Read the model definition and answer for the solid it produces. Units are mm, in the model's axes. A direction names the side the tool comes from. Coordinates: 2 decimals unless noted, no trailing zeros. Order: outer loops, then holes, each group sorted by start corner. A loop starts at its lowest first (then second) coordinate and runs counter-clockwise, first axis right, second up. Notation, with made-up numbers: M -12.75,41.5 L 8.25,41.5 A15 ccw 8.25,54.5 Z; hole C 11,-19 d4. An arc over 180 degrees is marked long. Write each question's results on one line, items separated by ' | '.
```python
from build123d import *

# Parameters (mm, degrees)
PCB_DEPTH                       = 1.6
SKETCH2_W                       = 2
SKETCH2_H                       = 30
BODY00_DEPTH                    = 0.4
SKETCH3_W                       = 80.5
SKETCH3_H                       = 54.92
BODY01_DEPTH                    = 4.2
SKETCH4_W                       = 6
SKETCH4_H                       = 12
UNDER00_DEPTH                   = 5
SKETCH5_W                       = 15
SKETCH5_H                       = 11.5
UNDER01_DEPTH                   = 5.6
SKETCH6_W                       = 33.02
SKETCH6_H                       = 5.08
UNDER02_DEPTH                   = 8.5
SKETCH7_R                       = 2.5
SIDE0_AUDIO_JACK_NOSE_DEPTH     = 2.5
SKETCH8_R                       = 1.75
SIDEBORE0_AUDIO_JACK_NOSE_DEPTH = 2.5
SKETCH9_W                       = 14
SKETCH9_H                       = 4.5
CUT00_DEPTH                     = 11
SKETCH10_W                      = 1
SKETCH10_H                      = 1
CUT01_DEPTH                     = 8.5
SKETCH11_W                      = 73.44
SKETCH11_H                      = 48.96
CUT02_DEPTH                     = 0.2
SKETCH12_R                      = 1.375
HOLES_DEPTH                     = 1.6


with BuildPart() as part:
    # Sketch1 → PCB (new body)
    with BuildSketch(Plane.XY):
        with BuildLine():
            Line((1, 0), (84.42, 0))
            ThreePointArc((84.42, 0), (85.127106781, 0.292893219), (85.42, 1))
            Line((85.42, 1), (85.42, 54.92))
            ThreePointArc((85.42, 54.92), (85.127106781, 55.627106781), (84.42, 55.92))
            Line((84.42, 55.92), (1, 55.92))
            ThreePointArc((1, 55.92), (0.292893219, 55.627106781), (0, 54.92))
            Line((0, 54.92), (0, 1))
            ThreePointArc((0, 1), (0.292893219, 0.292893219), (1, 0))
        make_face()
    extrude(amount=PCB_DEPTH)

    # Sketch2 → Body00 (add)
    with BuildSketch(Plane.XY.offset(1.6)):
        with Locations((82.3, 35)):
            Rectangle(SKETCH2_W, SKETCH2_H)
    extrude(amount=BODY00_DEPTH)

    # Sketch3 → Body01 (add)
    with BuildSketch(Plane.XY.offset(1.6)):
        with Locations((40.75, 27.96)):
            Rectangle(SKETCH3_W, SKETCH3_H)
    extrude(amount=BODY01_DEPTH)

    # Sketch4 → Under00 (add)
    with BuildSketch(Plane.XY):
        with Locations((53.5, 6)):
            Rectangle(SKETCH4_W, SKETCH4_H)
    extrude(amount=-UNDER00_DEPTH)

    # Sketch5 → Under01 (add)
    with BuildSketch(Plane.XY):
        with Locations((32, 5.25)):
            Rectangle(SKETCH5_W, SKETCH5_H)
    extrude(amount=-UNDER01_DEPTH)

    # Sketch6 → Under02 (add)
    with BuildSketch(Plane.XY):
        with Locations((23.61, 52.5)):
            Rectangle(SKETCH6_W, SKETCH6_H)
    extrude(amount=-UNDER02_DEPTH)

    # Sketch7 → Side0_Audio_jack_nose (add)
    with BuildSketch(Plane(origin=(0, 0, 0), x_dir=(1, 0, 0), z_dir=(0, 1, 0))):
        with Locations(Location((53.5, 2.5, 0), (0, 0, 270))):
            Circle(SKETCH7_R)
    extrude(amount=-SIDE0_AUDIO_JACK_NOSE_DEPTH)

    # Sketch8 → SideBore0_Audio_jack_nose (cut)
    with BuildSketch(Plane(origin=(0, 0, 0), x_dir=(1, 0, 0), z_dir=(0, 1, 0))):
        with Locations(Location((53.5, 2.5, 0), (0, 0, 270))):
            Circle(SKETCH8_R)
    extrude(amount=-SIDEBORE0_AUDIO_JACK_NOSE_DEPTH, mode=Mode.SUBTRACT)

    # Sketch9 → Cut00 (cut)
    with BuildSketch(Plane(origin=(0, 10.5, 0), x_dir=(1, 0, 0), z_dir=(0, 1, 0))):
        with Locations((32, 2.8)):
            Rectangle(SKETCH9_W, SKETCH9_H)
    extrude(amount=-CUT00_DEPTH, mode=Mode.SUBTRACT)

    # Sketch10 → Cut01 (cut)
    with BuildSketch(Plane.XY):
        with Locations((8.37, 51.23)):
            Rectangle(SKETCH10_W, SKETCH10_H)
        with Locations((8.37, 53.77)):
            Rectangle(SKETCH10_W, SKETCH10_H)
        with Locations((10.91, 51.23)):
            Rectangle(SKETCH10_W, SKETCH10_H)
        with Locations((10.91, 53.77)):
            Rectangle(SKETCH10_W, SKETCH10_H)
        with Locations((13.45, 51.23)):
            Rectangle(SKETCH10_W, SKETCH10_H)
        with Locations((13.45, 53.77)):
            Rectangle(SKETCH10_W, SKETCH10_H)
        with Locations((15.99, 51.23)):
            Rectangle(SKETCH10_W, SKETCH10_H)
        with Locations((15.99, 53.77)):
            Rectangle(SKETCH10_W, SKETCH10_H)
        with Locations((18.53, 51.23)):
            Rectangle(SKETCH10_W, SKETCH10_H)
        with Locations((18.53, 53.77)):
            Rectangle(SKETCH10_W, SKETCH10_H)
        with Locations((21.07, 51.23)):
            Rectangle(SKETCH10_W, SKETCH10_H)
        with Locations((21.07, 53.77)):
            Rectangle(SKETCH10_W, SKETCH10_H)
        with Locations((23.61, 51.23)):
            Rectangle(SKETCH10_W, SKETCH10_H)
        with Locations((23.61, 53.77)):
            Rectangle(SKETCH10_W, SKETCH10_H)
        with Locations((26.15, 51.23)):
            Rectangle(SKETCH10_W, SKETCH10_H)
        with Locations((26.15, 53.77)):
            Rectangle(SKETCH10_W, SKETCH10_H)
        with Locations((28.69, 51.23)):
            Rectangle(SKETCH10_W, SKETCH10_H)
        with Locations((28.69, 53.77)):
            Rectangle(SKETCH10_W, SKETCH10_H)
        with Locations((31.23, 51.23)):
            Rectangle(SKETCH10_W, SKETCH10_H)
        with Locations((31.23, 53.77)):
            Rectangle(SKETCH10_W, SKETCH10_H)
        with Locations((33.77, 51.23)):
            Rectangle(SKETCH10_W, SKETCH10_H)
        with Locations((33.77, 53.77)):
            Rectangle(SKETCH10_W, SKETCH10_H)
        with Locations((36.31, 51.23)):
            Rectangle(SKETCH10_W, SKETCH10_H)
        with Locations((36.31, 53.77)):
            Rectangle(SKETCH10_W, SKETCH10_H)
        with Locations((38.85, 51.23)):
            Rectangle(SKETCH10_W, SKETCH10_H)
        with Locations((38.85, 53.77)):
            Rectangle(SKETCH10_W, SKETCH10_H)
    extrude(amount=-CUT01_DEPTH, mode=Mode.SUBTRACT)

    # Sketch11 → Cut02 (cut)
    with BuildSketch(Plane.XY.offset(5.8)):
        with Locations((40, 27.96)):
            Rectangle(SKETCH11_W, SKETCH11_H)
    extrude(amount=-CUT02_DEPTH, mode=Mode.SUBTRACT)

    # Sketch12 → Holes (cut)
    with BuildSketch(Plane.XY.offset(1.6)):
        with Locations((3.5, 3.5)):
            Circle(SKETCH12_R)
        with Locations((3.5, 52.5)):
            Circle(SKETCH12_R)
        with Locations((61.5, 3.5)):
            Circle(SKETCH12_R)
        with Locations((61.5, 52.5)):
            Circle(SKETCH12_R)
    extrude(amount=-HOLES_DEPTH, mode=Mode.SUBTRACT)


solid = part.part
```
(1) The mould has two halves that part along Y. Classify faces 6 (the flat face through (32, 5, -0.55)), 7 (the flat face through (23, 49.96, -4)), 8 (the flat face through (52, -2.5, -1)): pulls with the +Y half, pulls with the -Y half, needs draft (parallel to the pull), parting line crosses it, or undercut.
Conclusion:
face 6: needs draft | face 7: undercut | face 8: pulls with the -Y half
(2) The part is cut by section D-D, the plane y = 23.5. Write down the section's boundary in (x, z).
Conclusion:
outline: M 0,0 L 85.42,0 L 85.42,1.6 L 83.3,1.6 L 83.3,2 L 81.3,2 L 81.3,1.6 L 81,1.6 L 81,5.8 L 76.72,5.8 L 76.72,5.6 L 3.28,5.6 L 3.28,5.8 L 0.5,5.8 L 0.5,1.6 L 0,1.6 Z
(3) Given pin 1 (0.8 mm diameter, centred on x = 11, z = -4.5, fed in from -Y); pin 2 (1.5 mm diameter, centred on x = 24, y = 4, fed in from -Z); pin 3 (2 mm diameter, centred on x = 51, z = -4, fed in from +Y); pin 4 (4 mm diameter, centred on y = 7.5, z = -1.5, fed in from +X), each flat-ended and moving along its own axis, determine where each tip first touches the part or whether it passes through.
Conclusion:
pin 1: y = 49.96 | pin 2: z = -5.6 | pin 3: y = 12 | pin 4: x = 85.42
(4) The part is cut by section C-C, the plane z = -2.5. Count the separate pieces of the cut face and the enclosed holes in it, then the cut area to 3 significant figures.
Conclusion:
separate pieces: 3 | enclosed holes: 26 | area: 236 mm²
(5) The part is cut by section A-A, the plane y = 8.5. Write down the section's boundary in (x, z).
Conclusion:
outline: M 0,0 L 24.5,0 L 24.5,-5.6 L 39.5,-5.6 L 39.5,0 L 50.5,0 L 50.5,-5 L 56.5,-5 L 56.5,0 L 85.42,0 L 85.42,1.6 L 81,1.6 L 81,5.8 L 76.72,5.8 L 76.72,5.6 L 3.28,5.6 L 3.28,5.8 L 0.5,5.8 L 0.5,1.6 L 0,1.6 Z; hole M 25,-5.05 L 39,-5.05 L 39,-0.55 L 25,-0.55 Z
(6) The part is cut by section B-B, the plane x = 78.5. Write down the section's boundary in (y, z).
Conclusion:
outline: M 0,0 L 55.92,0 L 55.92,1.6 L 55.42,1.6 L 55.42,5.8 L 0.5,5.8 L 0.5,1.6 L 0,1.6 Z
(7) For faces 1 (the flat face through (82, 35, 2)), 2 (the flat face through (40, 55.42, 4)), 3 (the flat face through (23, 55.04, -4)), 4 (the flat face through (7.1, 52, -4)), 5 (the flat face through (3, 4, 1.6)), determine the directions among +Z, -Z, +X, -X, +Y, -Y from which every point of the face is accessible in a straight line to the end or side of a thin tool.
Conclusion:
face 1: +Z, +X, +Y, -Y | face 2: +Z, +X, -X, +Y | face 3: -Z, +X, -X, +Y | face 4: -Z, -X, +Y, -Y | face 5: -Z
(8) Straight lines are drawn through the part: line 1 (Y direction, x = 36, z = -2); line 2 (Y direction, x = 3.5, z = 1) (3 decimals); line 3 (Y direction, x = 38, z = -3.75). For each, find the intervals that lie inside material, in ascending order.
Conclusion:
line 1: 10.5 to 11, 49.96 to 50.73, 51.73 to 53.27, 54.27 to 55.04 | line 2: 0 to 2.125, 4.875 to 51.125, 53.875 to 55.92 | line 3: 10.5 to 11, 49.96 to 55.04
